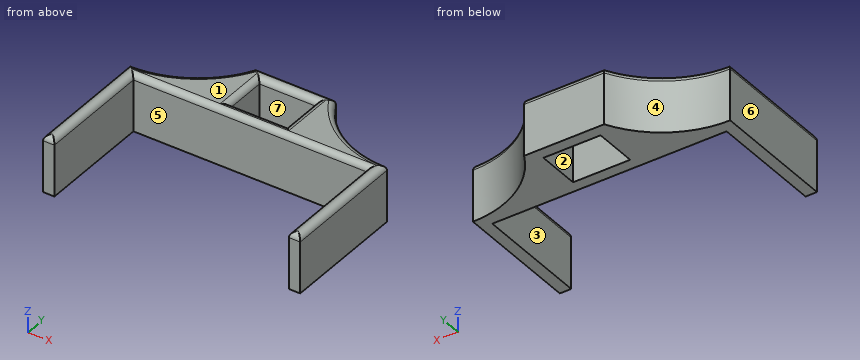
```python
from build123d import *

# Parameters (mm, degrees)
F0_W         = 10
F0_H         = 7.5
F1_DEPTH     = 10
F2_T1_DEPTH  = 26.9846032165
F2_T3_DEPTH  = 7
F2_T5_DEPTH  = 22.5
F2_T7_DEPTH  = 41
F2_T9_DEPTH  = 7
F2_T11_DEPTH = 19
F2_T13_DEPTH = 7.5
F2_T15_DEPTH = 10
F2_T18_ANGLE = 79.4810617097
F2_T20_ANGLE = 79.4810617097
F2_T25_DEPTH = 25
F2_T29_DEPTH = 43.5
F2_T36_DEPTH = 43.5
F2_T40_DEPTH = 25
F2_T47_DEPTH = 10
F2_T51_DEPTH = 12.5
F2_T58_DEPTH = 10
F2_T62_DEPTH = 12.5
F2_T69_DEPTH = 12.5
F2_T73_DEPTH = 10
F2_T80_DEPTH = 10
F2_T84_DEPTH = 12.5


# Not quite as in the source:
# - a fillet or chamfer that OpenCascade refuses, or shapes differently, is made with other operations: its cross-section is extruded or revolved along the edge and cut away or added


with BuildPart() as f1:
    # F0 (on Top) → F1 (new body)
    with BuildSketch(Plane.XY):
        with BuildLine():
            Line((0, 34.8731837149), (41, 34.8731837149))
            Line((41, 34.8731837149), (41, 14.8731837149))
            Line((41, 14.8731837149), (43, 14.8731837149))
            Line((43, 14.8731837149), (43, 36.8577869315))
            ThreePointArc((43, 36.8577869315), (33.9101705187, 39.4217493566), (27.5, 46.3577869315))
            Line((27.5, 46.3577869315), (13.5, 46.3577869315))
            ThreePointArc((13.5, 46.3577869315), (7.0898294813, 39.4217493566), (-2, 36.8577869315))
            Line((-2, 36.8577869315), (-2, 14.8731837149))
            Line((-2, 14.8731837149), (0, 14.8731837149))
            Line((0, 14.8731837149), (0, 34.8731837149))
        make_face()
        with Locations((20.5, 40.6077869315)):
            Rectangle(F0_W, F0_H, mode=Mode.SUBTRACT)
    extrude(amount=F1_DEPTH)

    # F2: fillet of radius 1 on 14 edges, made by hand

    # F2_s2 → F2_t1 (cut)
    with BuildSketch(Plane.XZ.offset(-39.3577869315)):
        with BuildLine():
            ThreePointArc((-2, 9), (-1.7071067812, 9.7071067812), (-1, 10))
            Line((-1, 10), (-2, 10))
            Line((-2, 10), (-2, 9))
        make_face()
        with BuildLine():
            ThreePointArc((43, 9), (42.7071067812, 9.7071067812), (42, 10))
            Line((42, 10), (43, 10))
            Line((43, 10), (43, 9))
        make_face()
    extrude(amount=F2_T1_DEPTH, mode=Mode.SUBTRACT)

    # F2_s4 → F2_t3 (cut)
    with BuildSketch(Plane.YZ.offset(-4.5)):
        with BuildLine():
            ThreePointArc((14.8731837149, 9), (15.1660769337, 9.7071067812), (15.8731837149, 10))
            Line((15.8731837149, 10), (14.8731837149, 10))
            Line((14.8731837149, 10), (14.8731837149, 9))
        make_face()
    extrude(amount=F2_T3_DEPTH, mode=Mode.SUBTRACT)

    # F2_s6 → F2_t5 (cut)
    with BuildSketch(Plane.XZ.offset(-34.8731837149)):
        with BuildLine():
            ThreePointArc((0, 9), (-0.2928932188, 9.7071067812), (-1, 10))
            Line((-1, 10), (0, 10))
            Line((0, 10), (0, 9))
        make_face()
        with BuildLine():
            ThreePointArc((41, 9), (41.2928932188, 9.7071067812), (42, 10))
            Line((42, 10), (41, 10))
            Line((41, 10), (41, 9))
        make_face()
    extrude(amount=F2_T5_DEPTH, mode=Mode.SUBTRACT)

    # F2_s8 → F2_t7 (cut)
    with BuildSketch(Plane.YZ):
        with BuildLine():
            ThreePointArc((34.8731837149, 9), (35.1660769337, 9.7071067812), (35.8731837149, 10))
            Line((35.8731837149, 10), (34.8731837149, 10))
            Line((34.8731837149, 10), (34.8731837149, 9))
        make_face()
    extrude(amount=F2_T7_DEPTH, mode=Mode.SUBTRACT)

    # F2_s10 → F2_t9 (cut)
    with BuildSketch(Plane.YZ.offset(38.5)):
        with BuildLine():
            ThreePointArc((14.8731837149, 9), (15.1660769337, 9.7071067812), (15.8731837149, 10))
            Line((15.8731837149, 10), (14.8731837149, 10))
            Line((14.8731837149, 10), (14.8731837149, 9))
        make_face()
    extrude(amount=F2_T9_DEPTH, mode=Mode.SUBTRACT)

    # F2_s12 → F2_t11 (cut)
    with BuildSketch(Plane.YZ.offset(11)):
        with BuildLine():
            ThreePointArc((46.3577869315, 9), (46.0648937127, 9.7071067812), (45.3577869315, 10))
            Line((45.3577869315, 10), (46.3577869315, 10))
            Line((46.3577869315, 10), (46.3577869315, 9))
        make_face()
    extrude(amount=F2_T11_DEPTH, mode=Mode.SUBTRACT)

    # F2_s14 → F2_t13 (cut)
    with BuildSketch(Plane.XZ.offset(-44.3577869315)):
        with BuildLine():
            ThreePointArc((25.5, 9), (25.7928932188, 9.7071067812), (26.5, 10))
            Line((26.5, 10), (25.5, 10))
            Line((25.5, 10), (25.5, 9))
        make_face()
        with BuildLine():
            ThreePointArc((15.5, 9), (15.2071067812, 9.7071067812), (14.5, 10))
            Line((14.5, 10), (15.5, 10))
            Line((15.5, 10), (15.5, 9))
        make_face()
    extrude(amount=F2_T13_DEPTH, mode=Mode.SUBTRACT)

    # F2_s16 → F2_t15 (cut)
    with BuildSketch(Plane.YZ.offset(15.5)):
        with BuildLine():
            ThreePointArc((36.8577869315, 9), (36.5648937127, 9.7071067812), (35.8577869315, 10))
            Line((35.8577869315, 10), (36.8577869315, 10))
            Line((36.8577869315, 10), (36.8577869315, 9))
        make_face()
        with BuildLine():
            ThreePointArc((44.3577869315, 9), (44.6506801503, 9.7071067812), (45.3577869315, 10))
            Line((45.3577869315, 10), (44.3577869315, 10))
            Line((44.3577869315, 10), (44.3577869315, 9))
        make_face()
    extrude(amount=F2_T15_DEPTH, mode=Mode.SUBTRACT)

    # F2_s17 → F2_t18 (revolve, cut)
    with BuildSketch(Plane(origin=(16.3105725922, 48.0350676987, 0), x_dir=(0, 0, 1), z_dir=(0.3215254447, 0.9469009391, 0))):
        with BuildLine():
            ThreePointArc((9, -1.9426318697), (9.7071067812, -1.6497386509), (10, -0.9426318697))
            Line((10, -0.9426318697), (10, -1.9426318697))
            Line((10, -1.9426318697), (9, -1.9426318697))
        make_face()
    revolve(axis=Axis((-2, 54.2525237736, 10), (0, 0, -1)), revolution_arc=F2_T18_ANGLE, mode=Mode.SUBTRACT)

    # F2_s19 → F2_t20 (revolve, cut)
    with BuildSketch(Plane(origin=(49.8093527962, 7.2098207335, 0), x_dir=(0, 0, 1), z_dir=(0.9896857587, 0.1432553627, 0))):
        with BuildLine():
            ThreePointArc((9, -30.138232714), (9.7071067812, -29.8453394951), (10, -29.138232714))
            Line((10, -29.138232714), (10, -30.138232714))
            Line((10, -30.138232714), (9, -30.138232714))
        make_face()
    revolve(axis=Axis((43, 54.2525237736, 10), (0, 0, -1)), revolution_arc=F2_T20_ANGLE, mode=Mode.SUBTRACT)


with BuildPart() as f2_tool23:
    # F2_s24 → F2_t25 (new body)
    with BuildSketch(Plane.XZ.offset(-12.3731837149)):
        with BuildLine():
            ThreePointArc((0, 9), (-0.2928932188, 9.7071067812), (-1, 10))
            Line((-1, 10), (0, 10))
            Line((0, 10), (0, 9))
        make_face()
    extrude(amount=-F2_T25_DEPTH)

    split(bisect_by=Plane.XZ.offset(-34.8731837149), keep=Keep.BOTTOM)


with BuildPart() as f2_tool27:
    # F2_s28 → F2_t29 (new body)
    with BuildSketch(Plane.YZ.offset(-2.5)):
        with BuildLine():
            ThreePointArc((34.8731837149, 9), (35.1660769337, 9.7071067812), (35.8731837149, 10))
            Line((35.8731837149, 10), (34.8731837149, 10))
            Line((34.8731837149, 10), (34.8731837149, 9))
        make_face()
    extrude(amount=F2_T29_DEPTH)

    split(bisect_by=Plane.YZ, keep=Keep.BOTTOM)


with BuildPart() as f2_tool23_1:
    add(f2_tool23.part)

    # F2_t31: intersect F2_tool27
    add(f2_tool27.part, mode=Mode.INTERSECT)


with BuildPart() as f1_1:
    add(f1.part)

    # F2_t21: cut F2_tool23
    add(f2_tool23_1.part, mode=Mode.SUBTRACT)


with BuildPart() as f2_tool34:
    # F2_s35 → F2_t36 (new body)
    with BuildSketch(Plane.YZ):
        with BuildLine():
            ThreePointArc((34.8731837149, 9), (35.1660769337, 9.7071067812), (35.8731837149, 10))
            Line((35.8731837149, 10), (34.8731837149, 10))
            Line((34.8731837149, 10), (34.8731837149, 9))
        make_face()
    extrude(amount=F2_T36_DEPTH)

    split(bisect_by=Plane.YZ.offset(41), keep=Keep.TOP)


with BuildPart() as f2_tool38:
    # F2_s39 → F2_t40 (new body)
    with BuildSketch(Plane.XZ.offset(-37.3731837149)):
        with BuildLine():
            ThreePointArc((41, 9), (41.2928932188, 9.7071067812), (42, 10))
            Line((42, 10), (41, 10))
            Line((41, 10), (41, 9))
        make_face()
    extrude(amount=F2_T40_DEPTH)

    split(bisect_by=Plane.XZ.offset(-34.8731837149), keep=Keep.BOTTOM)


with BuildPart() as f2_tool34_1:
    add(f2_tool34.part)

    # F2_t42: intersect F2_tool38
    add(f2_tool38.part, mode=Mode.INTERSECT)


with BuildPart() as f1_2:
    add(f1_1.part)

    # F2_t32: cut F2_tool34
    add(f2_tool34_1.part, mode=Mode.SUBTRACT)


with BuildPart() as f2_tool45:
    # F2_s46 → F2_t47 (new body)
    with BuildSketch(Plane.XZ.offset(-46.8577869315)):
        with BuildLine():
            ThreePointArc((25.5, 9), (25.7928932188, 9.7071067812), (26.5, 10))
            Line((26.5, 10), (25.5, 10))
            Line((25.5, 10), (25.5, 9))
        make_face()
    extrude(amount=F2_T47_DEPTH)

    split(bisect_by=Plane.XZ.offset(-44.3577869315), keep=Keep.BOTTOM)


with BuildPart() as f2_tool49:
    # F2_s50 → F2_t51 (new body)
    with BuildSketch(Plane.YZ.offset(15.5)):
        with BuildLine():
            ThreePointArc((44.3577869315, 9), (44.6506801503, 9.7071067812), (45.3577869315, 10))
            Line((45.3577869315, 10), (44.3577869315, 10))
            Line((44.3577869315, 10), (44.3577869315, 9))
        make_face()
    extrude(amount=F2_T51_DEPTH)

    split(bisect_by=Plane.YZ.offset(25.5), keep=Keep.TOP)


with BuildPart() as f2_tool45_1:
    add(f2_tool45.part)

    # F2_t53: intersect F2_tool49
    add(f2_tool49.part, mode=Mode.INTERSECT)


with BuildPart() as f1_3:
    add(f1_2.part)

    # F2_t43: cut F2_tool45
    add(f2_tool45_1.part, mode=Mode.SUBTRACT)


with BuildPart() as f2_tool56:
    # F2_s57 → F2_t58 (new body)
    with BuildSketch(Plane.XZ.offset(-44.3577869315)):
        with BuildLine():
            ThreePointArc((25.5, 9), (25.7928932188, 9.7071067812), (26.5, 10))
            Line((26.5, 10), (25.5, 10))
            Line((25.5, 10), (25.5, 9))
        make_face()
    extrude(amount=F2_T58_DEPTH)

    split(bisect_by=Plane.XZ.offset(-36.8577869315), keep=Keep.TOP)


with BuildPart() as f2_tool60:
    # F2_s61 → F2_t62 (new body)
    with BuildSketch(Plane.YZ.offset(28)):
        with BuildLine():
            ThreePointArc((36.8577869315, 9), (36.5648937127, 9.7071067812), (35.8577869315, 10))
            Line((35.8577869315, 10), (36.8577869315, 10))
            Line((36.8577869315, 10), (36.8577869315, 9))
        make_face()
    extrude(amount=-F2_T62_DEPTH)

    split(bisect_by=Plane.YZ.offset(25.5), keep=Keep.TOP)


with BuildPart() as f2_tool56_1:
    add(f2_tool56.part)

    # F2_t64: intersect F2_tool60
    add(f2_tool60.part, mode=Mode.INTERSECT)


with BuildPart() as f1_4:
    add(f1_3.part)

    # F2_t54: cut F2_tool56
    add(f2_tool56_1.part, mode=Mode.SUBTRACT)


with BuildPart() as f2_tool67:
    # F2_s68 → F2_t69 (new body)
    with BuildSketch(Plane.YZ.offset(25.5)):
        with BuildLine():
            ThreePointArc((36.8577869315, 9), (36.5648937127, 9.7071067812), (35.8577869315, 10))
            Line((35.8577869315, 10), (36.8577869315, 10))
            Line((36.8577869315, 10), (36.8577869315, 9))
        make_face()
    extrude(amount=-F2_T69_DEPTH)

    split(bisect_by=Plane.YZ.offset(15.5), keep=Keep.BOTTOM)


with BuildPart() as f2_tool71:
    # F2_s72 → F2_t73 (new body)
    with BuildSketch(Plane.XZ.offset(-34.3577869315)):
        with BuildLine():
            ThreePointArc((15.5, 9), (15.2071067812, 9.7071067812), (14.5, 10))
            Line((14.5, 10), (15.5, 10))
            Line((15.5, 10), (15.5, 9))
        make_face()
    extrude(amount=-F2_T73_DEPTH)

    split(bisect_by=Plane.XZ.offset(-36.8577869315), keep=Keep.TOP)


with BuildPart() as f2_tool67_1:
    add(f2_tool67.part)

    # F2_t75: intersect F2_tool71
    add(f2_tool71.part, mode=Mode.INTERSECT)


with BuildPart() as f1_5:
    add(f1_4.part)

    # F2_t65: cut F2_tool67
    add(f2_tool67_1.part, mode=Mode.SUBTRACT)


with BuildPart() as f2_tool78:
    # F2_s79 → F2_t80 (new body)
    with BuildSketch(Plane.XZ.offset(-36.8577869315)):
        with BuildLine():
            ThreePointArc((15.5, 9), (15.2071067812, 9.7071067812), (14.5, 10))
            Line((14.5, 10), (15.5, 10))
            Line((15.5, 10), (15.5, 9))
        make_face()
    extrude(amount=-F2_T80_DEPTH)

    split(bisect_by=Plane.XZ.offset(-44.3577869315), keep=Keep.BOTTOM)


with BuildPart() as f2_tool82:
    # F2_s83 → F2_t84 (new body)
    with BuildSketch(Plane.YZ.offset(13)):
        with BuildLine():
            ThreePointArc((44.3577869315, 9), (44.6506801503, 9.7071067812), (45.3577869315, 10))
            Line((45.3577869315, 10), (44.3577869315, 10))
            Line((44.3577869315, 10), (44.3577869315, 9))
        make_face()
    extrude(amount=F2_T84_DEPTH)

    split(bisect_by=Plane.YZ.offset(15.5), keep=Keep.BOTTOM)


with BuildPart() as f2_tool78_1:
    add(f2_tool78.part)

    # F2_t86: intersect F2_tool82
    add(f2_tool82.part, mode=Mode.INTERSECT)


with BuildPart() as f1_6:
    add(f1_5.part)

    # F2_t76: cut F2_tool78
    add(f2_tool78_1.part, mode=Mode.SUBTRACT)


solid = f1_6.part
```
Here's how the part is built. I have some questions about the finished solid (model axes, mm). Face numbers are marked on the shaded views. A direction names the side the tool comes from. Give positions to 0.01 mm unless a question says otherwise; leave off trailing zeros. Write each loop counter-clockwise with the first axis right and the second up, starting at its lowest first coordinate (ties: lowest second). Pieces come first, ordered by that corner, then holes. Notation, with made-up numbers: (-23, 50.25) -> (1, 50.25) arc R20 cw to (1, 57.25) -> close; hole circle Ø7 at (63.25, -23). An arc over 180 degrees is marked (long way). Write each question's results on one line, items separated by ' | '.
Item 1: If I drill on L1, parallel to X at y = 19, z = 6.75; L2, parallel to X at y = 20.5, z = 9.5; L3, parallel to Z at x = 24, y = 36, over which ranges is the centre line in solid material (lowest first)?
Output:
L1: x = -2 to 0, 41 to 43 | L2: x = -1.87 to -0.13, 41.13 to 42.87 | L3: z = 0 to 9.99
Item 2: Suppose I cut it at A-A on x = 19.5. Write out the boundary of the cut face in (y, z).
Output:
outline: (34.87, 0) -> (36.86, 0) -> (36.86, 9) arc R1 ccw to (35.87, 10) arc R1 ccw to (34.87, 9) -> close; (44.36, 0) -> (46.36, 0) -> (46.36, 9) arc R1 ccw to (44.36, 9) -> close
Item 3: Suppose I cut it at C-C on z = 2.5. Write out the boundary of the cut face in (x, y).
Output:
outline: (-2, 14.87) -> (0, 14.87) -> (0, 34.87) -> (41, 34.87) -> (41, 14.87) -> (43, 14.87) -> (43, 36.86) arc R17.39 cw to (27.5, 46.36) -> (13.5, 46.36) arc R17.39 cw to (-2, 36.86) -> close; hole (15.5, 36.86) -> (25.5, 36.86) -> (25.5, 44.36) -> (15.5, 44.36) -> close
Item 4: On a 3-axis mill with a long thin cutter (end or side, diameter ignored), from which of +Z, -Z, +X, -X, +Y, -Y can I reach the whole of each face in a straight line? I mean the marked faces 1, 2 and 3. Say none if no direction works.
Output:
face 1: +Z, +X, -X, +Y, -Y | face 2: +Z, -Z | face 3: +Z, -Z, -Y
Item 5: We'd pull the mould along Y, two halves only. Please class the marked faces 4, 5, 6 and 7: pulls with the +Y half, pulls with the -Y half, needs draft (parallel to the pull), parting line crosses it, or undercut.
Output:
face 4: pulls with the +Y half | face 5: pulls with the -Y half | face 6: needs draft | face 7: undercut
Item 6: For pin 1 Ø4 at (y, z) = (41, 6) entering from -X; pin 2 Ø6 at (y, z) = (42.5, 6.5) entering from +X; pin 3 Ø5 at (y, z) = (43, 4.5) entering from -X, each with a flat end and sliding along its axis, tell me the tip position at first contact or that it passes through.
Output:
pin 1: stops at x = 6.36 | pin 2: stops at x = 33.78 | pin 3: stops at x = 8.65
Item 7: Suppose I cut it at B-B on y = 26. Write out the boundary of the cut face in (x, z), plus the area to 3 significant figures.
Output:
outline: (-2, 0) -> (0, 0) -> (0, 9) arc R1 ccw to (-2, 9) -> close; (41, 0) -> (43, 0) -> (43, 9) arc R1 ccw to (41, 9) -> close | area: 39.1 mm^2
